Geometry: final body of the model. Coordinates: model frame, mm. A direction names the side the tool comes from. Give positions to 0.01 mm unless a question says otherwise; leave off trailing zeros. Order: outer loops, then holes, each group sorted by start corner. A loop starts at its lowest first (then second) coordinate and runs counter-clockwise, first axis right, second up. Notation, with made-up numbers: (33.5, 9) - (47.5, 9) arc R13 ccw to (47.5, 19) - close; hole circle Ø5 at (-32.75, 62.25). An arc over 180 degrees is marked (long way). One line per question, with ' | ' between items. Start each with the question number.
from build123d import *

# Parameters (mm, degrees)
HOLE_WIZARD_M41_D = 4.5


with BuildPart() as part:
    # Эскиз1 → Повернуть1 (revolve)
    with BuildSketch(Plane.XY, mode=Mode.PRIVATE) as revolve_1_sk:
        Polygon((5, 35), (22.5, 35), (22.5, 30), (12.5, 30), (12.5, 0), (5, 0), align=None)
    revolve(revolve_1_sk.sketch.rotate(Axis((0, 0, 0), (0, 1, 0)), 90), axis=Axis((0, 0, 0), (0, 1, 0)))

    # Отверстие с зазором M41 (through all)
    with Locations(Plane.XZ.offset(-30)):
        with Locations((-12.374368671, 12.374368671), (-12.374368671, -12.374368671), (12.374368671, -12.374368671), (12.374368671, 12.374368671)):
            Hole(HOLE_WIZARD_M41_D / 2)


solid = part.part
(1) Cut plane B-B, the plane z = 0. Return the cut outline in (x, y), plus the area to 3 significant figures.
(2) Cut plane C-C, the plane y = 32.5. Return the cut outline in (x, z), plus the area to 3 significant figures.
(3) Cut plane D-D, the plane y = 9. Return the cut outline in (x, z).
(4) Pull-direction query (X, two-part tool) for faces 1 (the flat face through (10, 30, -10)), 2 (the cylindrical face through (19.961, 32.465, -10.382)), 3 (the cylindrical face through (-14.52, 32.53, 13.05)); classes: +X half, -X half, draft (parallel to the pull), parting line (faces both ways), or undercut.
(5) Access query for faces 4 (the cylindrical face through (11.16, 32.53, 14.27)), 5 (the cylindrical face through (-3.755, 14.79, -11.923)). Directions: +Z, -Z, +X, -X, +Y, -Y. A direction counts if a zero-diameter tool reaches every point of the face in a straight line with its end or side. Return the directions, or none.
(6) Material intervals for line 1 along Y through (x, z) = (-21, -4.5); line 2 along X through (y, z) = (19, 0); line 3 along Z through (x, y) = (13, 32), sorted ascending. Write a range as from..to.
(7) Contact query for flat-ended pins moving along their axis: P1, Ø3, axis at x = 15, y = 6.5, coming from the -Z side; P2, Ø3, axis at y = 26.5, z = -4, coming from the +X side; P3, Ø22.5, axis at x = 0.5, z = -7, coming from the -Y side; P4, Ø1.5, axis at x = 10, y = 30.5, coming from the +Z side. Output: stop coordinate, or through.
(8) Cut plane A-A, the plane x = 0. Return the cut outline in (y, z).
Results are:
1) outline: (-22.5, 30) - (-12.5, 30) - (-12.5, 0) - (-5, 0) - (-5, 35) - (-22.5, 35) - close; (5, 0) - (12.5, 0) - (12.5, 30) - (22.5, 30) - (22.5, 35) - (5, 35) - close | area: 625 mm2
2) outline: circle Ø45 at (0, 0); hole circle Ø4.5 at (-12.37, -12.37); hole circle Ø4.5 at (-12.37, 12.37); hole circle Ø10 at (0, 0); hole circle Ø4.5 at (12.37, -12.37); hole circle Ø4.5 at (12.37, 12.37) | area: 1,450 mm2
3) outline: circle Ø25 at (0, 0); hole circle Ø10 at (0, 0)
4) face 1: draft | face 2: parting line | face 3: undercut
5) face 4: +Y, -Y | face 5: -Y
6) line 1: 30..35 | line 2: -12.5..-5, 5..12.5 | line 3: -18.36..-14.54, -10.21..10.21, 14.54..18.36
7) P1: through | P2: x = 12.25 | P3: y = 0 | P4: z = 20.51
8) outline: (0, -12.5) - (30, -12.5) - (30, -22.5) - (35, -22.5) - (35, -5) - (0, -5) - close; (0, 5) - (35, 5) - (35, 22.5) - (30, 22.5) - (30, 12.5) - (0, 12.5) - close
